Part model, mm, in its own coordinate system. A direction names the side the tool comes from. Coordinates: 2 decimals unless noted, no trailing zeros. Order: outer loops, then holes, each group sorted by start corner. A loop starts at its lowest first (then second) coordinate and runs counter-clockwise, first axis right, second up. Notation, with made-up numbers: M 43.25,-3.5 L 79.25,-3.5 A24 ccw 79.25,23.5 Z; hole C 18.5,65.25 d1. An arc over 180 degrees is marked long. Write item = value, one per line. Start each with the question number.
from build123d import *

# Parameters (mm, degrees)
F1_W     = 3
F1_H     = 20
F2_DEPTH = 15
F3_DEPTH = 3


with BuildPart() as f2:
    # F1 (on offset) → F2 (new body, through all)
    with BuildSketch(Plane.XZ.offset(15)):
        with Locations((78.5, 10)):
            Rectangle(F1_W, F1_H)
    extrude(amount=-F2_DEPTH)



with BuildPart() as f2b:
    # F1 (on offset) → F2, piece 2 (new body, through all)
    with BuildSketch(Plane.XZ.offset(15)):
        with Locations((-78.5, 10)):
            Rectangle(F1_W, F1_H)
    extrude(amount=-F2_DEPTH)


with BuildPart() as f2_1:
    add(f2.part)

    add(f2b.part)  # F3 merges F2b
    # F1 (on offset) → F3 (join)
    with BuildSketch(Plane.XZ.offset(15)):
        with BuildLine():
            Line((0, 5), (0, 0))
            Line((0, 0), (67, 0))
            Line((67, 0), (77, 0))
            Line((77, 0), (77, 20))
            Line((77, 20), (0, 20))
            Line((0, 20), (0, 15))
            Line((0, 15), (65, 15))
            ThreePointArc((65, 15), (68.5355339059, 13.5355339059), (70, 10))
            ThreePointArc((70, 10), (68.5355339059, 6.4644660941), (65, 5))
            Line((65, 5), (0, 5))
        make_face()
        with BuildLine():
            Line((-67, 10), (-67, 0))
            Line((-67, 0), (0, 0))
            Line((0, 0), (0, 5))
            ThreePointArc((0, 5), (-5, 10), (0, 15))
            Line((0, 15), (0, 20))
            Line((0, 20), (-67, 20))
            Line((-67, 20), (-67, 10))
        make_face()
        with BuildLine():
            ThreePointArc((-57, 10), (-62, 5), (-67, 10))
            ThreePointArc((-67, 10), (-62, 15), (-57, 10))
        make_face(mode=Mode.SUBTRACT)
        Polygon((-77, 20), (-77, 0), (-67, 0), (-67, 10), (-67, 20), align=None)
        with Locations((-78.5, 10)):
            Rectangle(F1_W, F1_H)
        with Locations((78.5, 10)):
            Rectangle(F1_W, F1_H)
    extrude(amount=F3_DEPTH)

    # F4: F2 across plane


with BuildPart() as f2_2:
    add(f2_1.part)
    add(f2_1.part.mirror(Plane.XZ))


solid = f2_2.part
Item 1: Cut at D-D, the plane z = 6.75. Write the cut outline in (x, y).
Item 2: Wall check: line 1 along Y through (x, z) = (-11, 9.25); line 2 along X through (y, z) = (-0.5, 9.25); line 3 along Z through (x, y) = (-62, 16.75). Give the ranges that are in metal, low to high. Write a range as [from, to].
Item 3: Cut at A-A, the plane x = 53.5. Write the cut outline in (y, z).
Item 4: Cut at B-B, the plane y = 9.5. Write the cut outline in (x, z), and give its area (3 significant figures).
Item 5: Pull direction Y, two halves, no side cores. Call faces 1 (the flat face through (-19, 18, 10)), 2 (the flat face through (-77, 0, 10)), 3 (the flat face through (32, 16, 15)): pulls with the +Y half, pulls with the -Y half, needs draft (parallel to the pull), parting line crosses it, or undercut.
Item 6: Cut at C-C, the plane z = 17.75. Write the cut outline in (x, y), and give its area (3 significant figures).
Item 7: 3-axis set-ups, long thin cutter, end or side, ignore diameter. For faces 4 (the flat face through (32, -16, 15)), 5 (the flat face through (-12, 16, 0)), 6 (the flat face through (-18, -15, 10)): which of +Z, -Z, +X, -X, +Y, -Y reach the whole face in a straight line?
Filled sheet:
q1.outline = M -80,-18 L -65.8,-18 L -65.8,-15 L -77,-15 L -77,15 L -65.8,15 L -65.8,18 L -80,18 Z; M -58.2,-18 L -3.8,-18 L -3.8,-15 L -58.2,-15 Z; M -58.2,15 L -3.8,15 L -3.8,18 L -58.2,18 Z; M 68.8,-18 L 80,-18 L 80,18 L 68.8,18 L 68.8,15 L 77,15 L 77,-15 L 68.8,-15 Z
q2.line_1 = [-18, -15], [15, 18]
q2.line_2 = [-80, -77], [77, 80]
q2.line_3 = [0, 5], [15, 20]
q3.outline = M -18,0 L -15,0 L -15,5 L -18,5 Z; M -18,15 L -15,15 L -15,20 L -18,20 Z; M 15,0 L 18,0 L 18,5 L 15,5 Z; M 15,15 L 18,15 L 18,20 L 15,20 Z
q4.outline = M -80,0 L -77,0 L -77,20 L -80,20 Z; M 77,0 L 80,0 L 80,20 L 77,20 Z
q4.area = 120 mm2
q5.face_1 = pulls with the +Y half
q5.face_2 = undercut
q5.face_3 = needs draft
q6.outline = M -80,-18 L 80,-18 L 80,18 L -80,18 Z; hole M -77,-15 L 77,-15 L 77,15 L -77,15 Z
q6.area = 1,140 mm2
q7.face_4 = +Y, -Y
q7.face_5 = -Z, +X, -X, +Y, -Y
q7.face_6 = +Z, -Z
